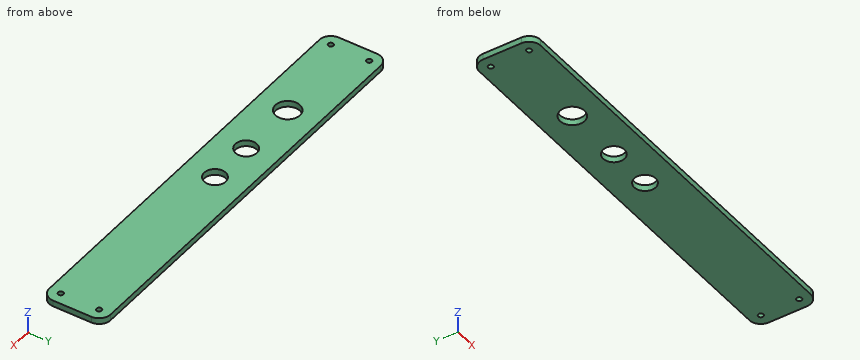
```python
from build123d import *

# Parameters (mm, degrees)
SKETCH_1_W          = 40
SKETCH_1_H          = 275
EXTRUDE_1_DEPTH     = 4
SKETCH_2_R          = 8
SKETCH_2_R_2        = 7
CUT_EXTRUDE_1_DEPTH = 5
HOLE_WIZARD_M3_1_D  = 3.4
FILLET_1_R          = 7.5


with BuildPart() as part:
    # ｽｹｯﾁ1 → ﾎﾞｽ - 押し出し1 (new body)
    with BuildSketch(Plane(origin=(0, 0, 0), x_dir=(0, 1, 0), z_dir=(0, 0, 1))):
        with Locations((20, 137.5)):
            Rectangle(SKETCH_1_W, SKETCH_1_H)
    extrude(amount=EXTRUDE_1_DEPTH)

    # ｽｹｯﾁ2 → ｶｯﾄ - 押し出し1 (cut, through all)
    with BuildSketch(Plane.XY.offset(4)):
        with Locations((-207.5, 20)):
            Circle(SKETCH_2_R)
        with Locations((-167.5, 20)):
            Circle(SKETCH_2_R_2)
        with Locations((-137.5, 20)):
            Circle(SKETCH_2_R_2)
    extrude(amount=-CUT_EXTRUDE_1_DEPTH, mode=Mode.SUBTRACT)

    # M3 すきま穴1 (through all)
    with Locations(Plane.XY.offset(4)):
        with Locations((-267.5, 32.5), (-267.5, 7.5), (-7.5, 7.5), (-7.5, 32.5)):
            Hole(HOLE_WIZARD_M3_1_D / 2)

    # ﾌｨﾚｯﾄ1
    fillet_1_edges = [part.edges().sort_by_distance(p)[0] for p in [
        (-275, 0, 2),
        (-275, 40, 2),
        (0, 40, 2),
        (0, 0, 2),
    ]]
    fillet(fillet_1_edges, radius=FILLET_1_R)


solid = part.part
```
Read the model definition and answer for the solid it produces. Units are mm, in the model's axes. Coordinates: 2 decimals unless noted, no trailing zeros. Order: outer loops, then holes, each group sorted by start corner. A loop starts at its lowest first (then second) coordinate and runs counter-clockwise, first axis right, second up. Notation, with made-up numbers: (39, -31.5) - (71, -31.5) arc R7 cw to (71, -26.5) - close; hole circle Ø9 at (8, -5.75). An arc over 180 degrees is marked (long way). Answer as a JSON object with one key per item and string values. Group by question number.
Item 1: Section B-B (y = 20) is taken. Give the vertices of the cut face in (x, z).
Item 2: Consider probe 1 along Y at (x, z) = (-267.5, 0.8); probe 2 along X at (y, z) = (16.5, 1.4); probe 3 along Y at (x, z) = (-137.5, 2.5). Determine where each line is inside the solid, lowest interval first. Write a range as from..to.
Item 3: Flat-ended cylindrical pins translate along their axes: P1, Ø21, axis at x = -207.5, y = 20, coming from the +Z side; P2, Ø2, axis at y = 35.5, z = 2.5, coming from the +X side. Find the tip coordinate at first contact, or state that the pin passes through.
Item 4: Section C-C (z = 2.2) is taken. Give the vertices of the cut face in (x, y).
Item 5: Section A-A (x = -137.5) is taken. Give the vertices of the cut face in (y, z).
Results are:
{
 "1": {"outline": "(-275, 0) - (-215.5, 0) - (-215.5, 4) - (-275, 4) - close; (-199.5, 0) - (-174.5, 0) - (-174.5, 4) - (-199.5, 4) - close; (-160.5, 0) - (-144.5, 0) - (-144.5, 4) - (-160.5, 4) - close; (-130.5, 0) - (0, 0) - (0, 4) - (-130.5, 4) - close"},
 "2": {"probe 1": "y = 0..5.8, 9.2..30.8, 34.2..40", "probe 2": "x = -275..-214.69, -200.31..-173.56, -161.44..-143.56, -131.44..0", "probe 3": "y = 0..13, 27..40"},
 "3": {"P1": "stops at z = 4", "P2": "stops at x = -0.27"},
 "4": {"outline": "(-275, 7.5) arc R7.5 ccw to (-267.5, 0) - (-7.5, 0) arc R7.5 ccw to (0, 7.5) - (0, 32.5) arc R7.5 ccw to (-7.5, 40) - (-267.5, 40) arc R7.5 ccw to (-275, 32.5) - close; hole circle Ø3.4 at (-267.5, 7.5); hole circle Ø3.4 at (-267.5, 32.5); hole circle Ø16 at (-207.5, 20); hole circle Ø14 at (-167.5, 20); hole circle Ø14 at (-137.5, 20); hole circle Ø3.4 at (-7.5, 7.5); hole circle Ø3.4 at (-7.5, 32.5)"},
 "5": {"outline": "(0, 0) - (13, 0) - (13, 4) - (0, 4) - close; (27, 0) - (40, 0) - (40, 4) - (27, 4) - close"}
}
